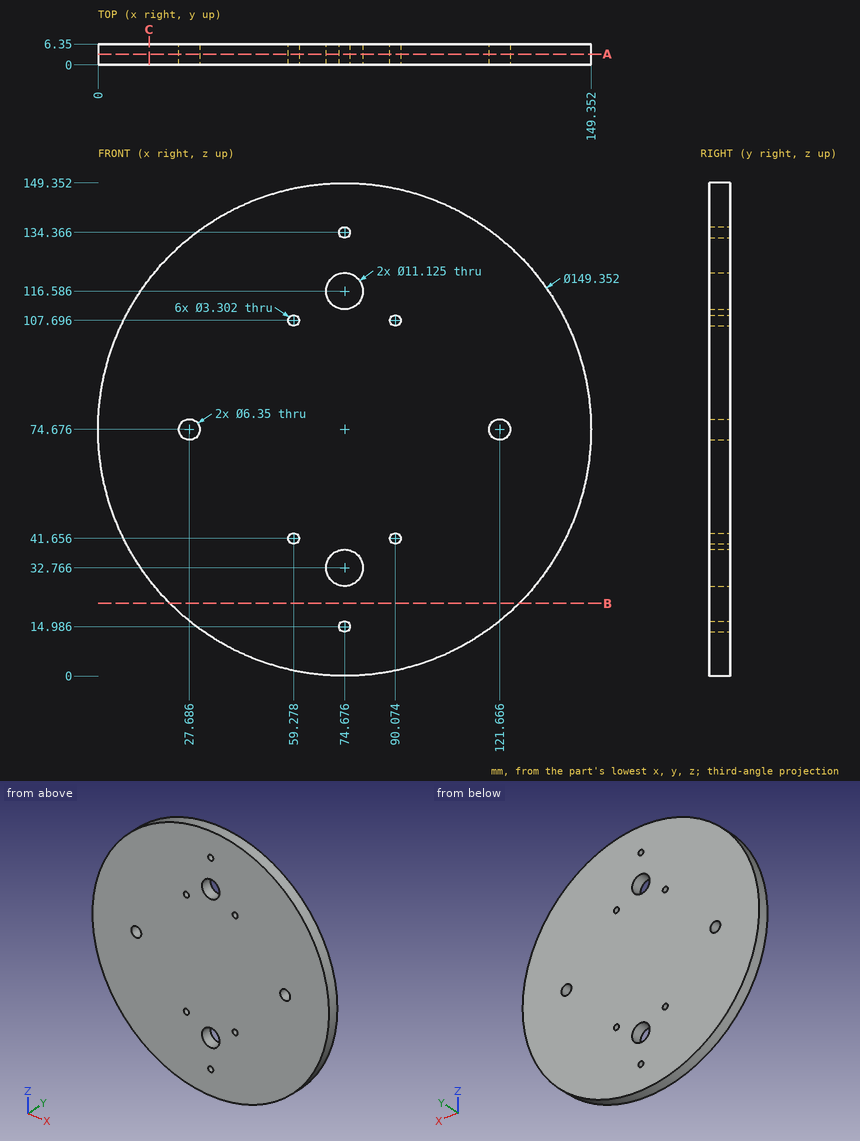
Could you check a few things on this drawing? It's one solid part, dimensions in mm from its lowest x, y, z. Round coordinates to 2 decimals unless told otherwise and drop trailing zeros. Order: outer loops, then holes, each group sorted by start corner. A loop starts at its lowest first (then second) coordinate and runs counter-clockwise, first axis right, second up. Notation, with made-up numbers: M 26,73 L 41,73 A19 ccw 41,102 Z; hole C 85.5,52.25 d6. An arc over 180 degrees is marked long. One line per question, with ' | ' between items. Start each with the question number.
(1) Suppose I cut it at A-A on y = 3.25. Count the separate pieces of the cut face and the enclosed holes in it, then the cut area to 3 significant figures.
(2) For P1, Ø3, axis at x = 74.676, z = 14.986, coming from the +Y side; P2, Ø4.5, axis at x = 90.07, z = 41.66, coming from the -Y side; P3, Ø3, axis at x = 129.5, y = 4.5, coming from the -Z side; P4, Ø1.5, axis at y = 2, z = 80.5, coming from the -X side, each with a flat end and sliding along its axis, tell me the tip position at first contact or that it passes through.
(3) Suppose I cut it at C-C on x = 15.5. List the corners of the cut face in (y, z) for me (3 decimals).
(4) Suppose I cut it at B-B on z = 22. List the corners of the cut face in (x, y) for me, then the cut area to 3 significant figures.
(5) Please list where these lines run through material, in increasing order: line 1 along X through (y, z) = (6, 41.5) (1 decimal); line 2 along X through (y, z) = (6.25, 40.5) (1 decimal); line 3 along Z through (x, y) = (60.5, 5) (1 decimal).
Geometry results:
1) separate pieces: 1 | enclosed holes: 10 | area: 17,200 mm²
2) P1: through | P2: y = 0 | P3: z = 22.4 | P4: x = 0.17
3) outline: M 0,29.127 L 6.35,29.127 L 6.35,120.225 L 0,120.225 Z
4) outline: M 21.74,0 L 127.61,0 L 127.61,6.35 L 21.74,6.35 Z | area: 672 mm²
5) line 1: 7.8 to 57.6, 60.9 to 88.4, 91.7 to 141.6 | line 2: 8.3 to 58.1, 60.5 to 88.9, 91.3 to 141.1 | line 3: 1.4 to 40.5, 42.8 to 106.6, 108.8 to 148
